from build123d import *

# Parameters (mm, degrees)
SKETCH1_R           = 5
BOSS_EXTRUDE1_DEPTH = 35
CUT_EXTRUDE1_REACH  = 28
SKETCH2_R           = 2


with BuildPart() as part:
    # Sketch1 → Boss-Extrude1 (new body)
    with BuildSketch(Plane.XY):
        Polygon((-7.376347734, 13), (-10.704853009, 8), (-19.287228785, 8), (-20, 6.929292346), (-20, -13), (-12.193167268, -13), (-10.704853009, -13), (-9.216538749, -11.511685741), (9.216538749, -11.511685741), (10.704853009, -13), (12.193167268, -13), (20, -13), (20, 6.929292346), (19.287228785, 8), (10.704853009, 8), (7.376347734, 13), align=None)
        Circle(SKETCH1_R, mode=Mode.SUBTRACT)
    extrude(amount=BOSS_EXTRUDE1_DEPTH)

    # Sketch2 → Cut-Extrude1 (cut, up to next)
    with BuildSketch(Plane.XZ.offset(13), mode=Mode.PRIVATE) as cut_extrude1_sk1:
        with Locations((-14, 28)):
            Circle(SKETCH2_R)
    cut_extrude1_tool1 = extrude(cut_extrude1_sk1.sketch, amount=-CUT_EXTRUDE1_REACH, mode=Mode.PRIVATE) & part.part
    add(cut_extrude1_tool1.solids().sort_by_distance((-14, -13, 28))[0], mode=Mode.SUBTRACT)
    # Sketch2 → Cut-Extrude1 (cut, up to next)
    with BuildSketch(Plane.XZ.offset(13), mode=Mode.PRIVATE) as cut_extrude1_sk2:
        with Locations((14, 28)):
            Circle(SKETCH2_R)
    cut_extrude1_tool2 = extrude(cut_extrude1_sk2.sketch, amount=-CUT_EXTRUDE1_REACH, mode=Mode.PRIVATE) & part.part
    add(cut_extrude1_tool2.solids().sort_by_distance((14, -13, 28))[0], mode=Mode.SUBTRACT)
    # Sketch2 → Cut-Extrude1 (cut, up to next)
    with BuildSketch(Plane.XZ.offset(13), mode=Mode.PRIVATE) as cut_extrude1_sk3:
        with Locations((14, 7)):
            Circle(SKETCH2_R)
    cut_extrude1_tool3 = extrude(cut_extrude1_sk3.sketch, amount=-CUT_EXTRUDE1_REACH, mode=Mode.PRIVATE) & part.part
    add(cut_extrude1_tool3.solids().sort_by_distance((14, -13, 7))[0], mode=Mode.SUBTRACT)
    # Sketch2 → Cut-Extrude1 (cut, up to next)
    with BuildSketch(Plane.XZ.offset(13), mode=Mode.PRIVATE) as cut_extrude1_sk4:
        with Locations((-14, 7)):
            Circle(SKETCH2_R)
    cut_extrude1_tool4 = extrude(cut_extrude1_sk4.sketch, amount=-CUT_EXTRUDE1_REACH, mode=Mode.PRIVATE) & part.part
    add(cut_extrude1_tool4.solids().sort_by_distance((-14, -13, 7))[0], mode=Mode.SUBTRACT)


solid = part.part
Source: CAD feature listing. Evaluate the final solid. Frame: model axes, mm. A direction names the side the tool comes from. Give positions to 0.01 mm unless a question says otherwise; leave off trailing zeros. Write each loop counter-clockwise with the first axis right and the second up, starting at its lowest first coordinate (ties: lowest second). Pieces come first, ordered by that corner, then holes. Notation, with made-up numbers: (87, 25) -> (98, 25) arc R30 cw to (98, 54) -> close; hole circle Ø11 at (75.5, -37.5). An arc over 180 degrees is marked (long way). Return JSON: item names as keys, results as strings. Group by question number.
1. Section A-A, the plane z = 28. Output: boundary loops of the cut face in (x, y), then the cut area to 3 significant figures.
2. Section B-B, the plane x = -14. Output: boundary loops of the cut face in (y, z), then the cut area to 3 significant figures.
3. Section C-C, the plane y = 0. Output: boundary loops of the cut face in (x, z), then the cut area to 4 significant figures.
4. Section D-D, the plane z = 32.5. Output: boundary loops of the cut face in (x, y), then the cut area to 3 significant figures.
5. Access query for faces 1 (the face through (15, 8, 17)), 2 (the face through (-20, -3, 17)), 3 (the face through (-9.971, -12.266, 17.255)). Directions: +Z, -Z, +X, -X, +Y, -Y. A direction counts if a zero-diameter tool reaches every point of the face in a straight line with its end or side. Return the directions, or none.
6. Material intervals for line 1 (Z direction, x = 14, y = -2.25); line 2 (Y direction, x = 6, z = 16.5); line 3 (Y direction, x = -16, z = 5.5), sorted ascending. Write a range as from..to.
7. Mould query, pull axis X, two halves, no side actions, for faces 4 (the face through (15, -13, 17)), 5 (the face through (20, -3, 17)), 6 (the face through (14, -3, 26)), 7 (the face through (-1.08, -4.88, 17.26)). Classes: +X half, -X half, draft (parallel to the pull), parting line (faces both ways), or undercut.
8. Pin query (flat end, axial travel): pin 1 Ø4.5 at (x, z) = (14, 7) entering from +Y; pin 2 Ø3 at (x, z) = (-10, 12) entering from +Y. Return the tip coordinate at first contact, or that it passes through.
Determined:
{
 "1": {"outline": "(-20, -13) -> (-16, -13) -> (-16, 8) -> (-19.29, 8) -> (-20, 6.93) -> close; (-12, -13) -> (-10.7, -13) -> (-9.22, -11.51) -> (9.22, -11.51) -> (10.7, -13) -> (12, -13) -> (12, 8) -> (10.7, 8) -> (7.38, 13) -> (-7.38, 13) -> (-10.7, 8) -> (-12, 8) -> close; (16, -13) -> (20, -13) -> (20, 6.93) -> (19.29, 8) -> (16, 8) -> close; hole circle Ø10 at (0, 0)", "area": "653 mm2"},
 "2": {"outline": "(-13, 0) -> (8, 0) -> (8, 5) -> (-13, 5) -> close; (-13, 9) -> (8, 9) -> (8, 26) -> (-13, 26) -> close; (-13, 30) -> (8, 30) -> (8, 35) -> (-13, 35) -> close", "area": "567 mm2"},
 "3": {"outline": "(-20, 0) -> (-5, 0) -> (-5, 35) -> (-20, 35) -> close; (5, 0) -> (20, 0) -> (20, 35) -> (5, 35) -> close; hole circle Ø4 at (-14, 7); hole circle Ø4 at (-14, 28); hole circle Ø4 at (14, 7); hole circle Ø4 at (14, 28)", "area": "1,000 mm2"},
 "4": {"outline": "(-20, -13) -> (-10.7, -13) -> (-9.22, -11.51) -> (9.22, -11.51) -> (10.7, -13) -> (20, -13) -> (20, 6.93) -> (19.29, 8) -> (10.7, 8) -> (7.38, 13) -> (-7.38, 13) -> (-10.7, 8) -> (-19.29, 8) -> (-20, 6.93) -> close; hole circle Ø10 at (0, 0)", "area": "821 mm2"},
 "5": {"face 1": "+Z, -Z, +X, +Y", "face 2": "+Z, -Z, -X, +Y, -Y", "face 3": "+Z, -Z, -Y"},
 "6": {"line 1": "z = 0..5, 9..26, 30..35", "line 2": "y = -11.51..13", "line 3": "y = -13..8"},
 "7": {"face 4": "draft", "face 5": "+X half", "face 6": "undercut", "face 7": "undercut"},
 "8": {"pin 1": "stops at y = 8", "pin 2": "stops at y = 11.31"}
}
